Autodesk Fusion 360 part; units mm, degrees
sketch "Sketch1" plane through (0, 0, 0) normal (0, 1, 0) x (1, 0, 0) in component "Limit Interrupter"
  line L0 (0, 0) -> (0, -7.014)
  line L1 (0, -7.014) -> (1.5, -7.014)
  line L2 (1.5, -7.014) -> (1.5, 0)
  line L3 (1.5, 0) -> (2.5, 0)
  line L4 (2.5, 0) -> (2.5, -8)
  line L5 (2.5, -8) -> (-1, -8)
  line L6 (-1, -8) -> (-1, 0)
  line L7 (-1, 0) -> (0, 0)
  line L8 (-1, -4.9804) -> (-7, -4.9804)
  line L9 (-7, -4.9804) -> (-7, -3.9804)
  line L10 (-7, -3.9804) -> (-1, -3.9804)
  dimension "d1" = 1
  dimension "d2" = 3.5
  dimension "d3" = 1.5
  dimension "d4" = 6
  dimension "d5" = 1
  dimension "d6" = 8
  dimension "d7" = 8
extrude "Extrude1" add sketch "Sketch1" along normal blind 10 in component "Limit Interrupter"
hole "Hole1" at (-3.7627, 5.2663, 4.9804) direction (0, 0, -1) diameter 1 depth 2 tip angle 118 in component "Limit Interrupter"
sketch "Sketch1 (2)" plane through (0, 0, 0) normal (0, -1, 0) x (1, 0, 0)
  line L0 (-7, 4.9804) -> (-7, 3.9804)
  line L1 (-7, 3.9804) -> (-1, 3.9804)
  line L2 (-1, 3.9804) -> (-1, 0)
  line L3 (-1, 0) -> (0, 0)
  line L4 (0, 0) -> (0, 7.014)
  line L5 (0, 7.014) -> (1.5, 7.014)
  line L6 (1.5, 7.014) -> (1.5, 0)
  line L7 (1.5, 0) -> (2.5, 0)
  line L8 (2.5, 0) -> (2.5, 8)
  line L9 (2.5, 8) -> (-1, 8)
  line L10 (-1, 8) -> (-1, 4.9804)
  line L11 (-1, 4.9804) -> (-7, 4.9804)
  line L12 (0, 0) -> (0.8, 0)
  line L13 (0.8, 0) -> (0.8, 7.014)
  line L14 (0.8, 7.014) -> (0, 7.014)
  dimension "d13" = 0.8
  dimension "d14" = 7.014
extrude "Extrude2" add sketch "Sketch1 (2)" against normal blind 0.8 contours L4 L5 L12 L13 L14 in component "Limit Interrupter"
component "Limit Interrupter" placed x (1, 0, 0) y (0, 1, 0) z (0, 0, 1) at (0, 0, 0)
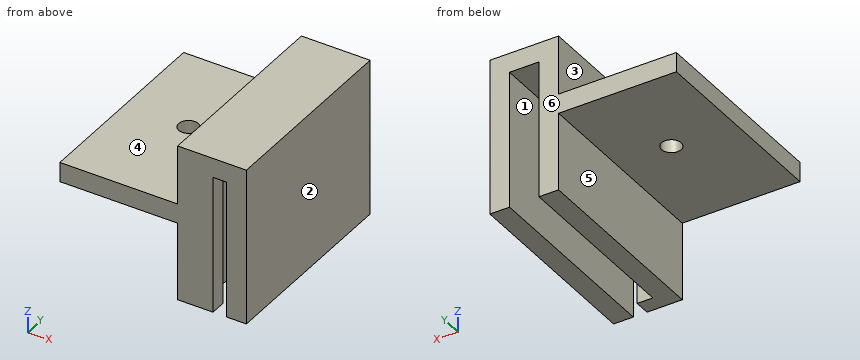
Geometry check sheet. Reference: the model listing, model coordinates, mm. Face numbers are marked on the shaded views. A direction names the side the tool comes from. Coordinates: 2 decimals unless noted, no trailing zeros. Order: outer loops, then holes, each group sorted by start corner. A loop starts at its lowest first (then second) coordinate and runs counter-clockwise, first axis right, second up. Notation, with made-up numbers: (44.25, 61.25) - (52.25, 61.25) arc R22 ccw to (52.25, 69.25) - close; hole circle Ø4 at (82.25, 83). An arc over 180 degrees is marked (long way). Answer in a Markdown table with one row per item. Add a question column.
1. Material ranges on L1, parallel to X at y = 2, z = 6; L2, parallel to X at y = 8.75, z = 4.5; L3, parallel to Z at x = -5.5, y = 2.25, recorded low to high. Write a range as [from, to].
2. Section check D-D (x = -5.5). Enter the section's corners in (y, z).
3. Draft check along X on the marked faces 1, 2 and 3. Enter one of: +X half, -X half, draft (parallel to the pull), parting line (faces both ways), or undercut.
4. Access from +Z, -Z, +X, -X, +Y, -Y to the whole of each face (thin tool, end or side, straight path). Record for the marked faces 4, 5 and 6.
5. Gauge pin test, flat ends, axial feed: pin 1 Ø2 at (x, y) = (-5, 2) entering from +Z; pin 2 Ø0.8 at (x, y) = (0.5, 6.5) entering from -Z. Record the tip position at first contact, or that the pin passes through.
6. Section check C-C (z = 3). Enter the section's corners in (x, y).
7. Section check B-B (y = 6.5). Enter the section's corners in (x, z), plus the area to 3 significant figures.
8. Section check A-A (z = 4.75). Enter the section's corners in (x, y).
Data:
| question | item | result |
|---|---|---|
| 1 | L1 | x = [-1, 0], [1.5, 2.5] |
| 1 | L2 | x = [-7, 0], [1.5, 2.5] |
| 1 | L3 | z = [3.98, 4.98] |
| 2 | outline | (0, 3.98) - (10, 3.98) - (10, 4.98) - (0, 4.98) - close |
| 3 | face 1 | undercut |
| 3 | face 2 | +X half |
| 3 | face 3 | -X half |
| 4 | face 4 | +Z, -X, +Y, -Y |
| 4 | face 5 | -Z, -X, +Y, -Y |
| 4 | face 6 | +Z, -Z, +X, -X, +Y |
| 5 | pin 1 | stops at z = 4.98 |
| 5 | pin 2 | stops at z = 7.01 |
| 6 | outline | (-1, 0) - (0.8, 0) - (0.8, 0.8) - (0, 0.8) - (0, 10) - (-1, 10) - close; (1.5, 0) - (2.5, 0) - (2.5, 10) - (1.5, 10) - close |
| 7 | outline | (-7, 3.98) - (-1, 3.98) - (-1, 0) - (0, 0) - (0, 7.01) - (1.5, 7.01) - (1.5, 0) - (2.5, 0) - (2.5, 8) - (-1, 8) - (-1, 4.98) - (-7, 4.98) - close |
| 7 | area | 23.5 mm² |
| 8 | outline | (-7, 0) - (0.8, 0) - (0.8, 0.8) - (0, 0.8) - (0, 10) - (-7, 10) - close; (1.5, 0) - (2.5, 0) - (2.5, 10) - (1.5, 10) - close; hole circle Ø1 at (-3.76, 5.27) |
